Autodesk Inventor part; units mm, degrees
ref_plane "YZ Plane" through (0, 0, 0) normal (1, 0, 0) x (0, 1, 0)
ref_plane "XZ Plane" through (0, 0, 0) normal (0, 1, 0) x (-1, 0, 0)
ref_plane "XY Plane" through (0, 0, 0) normal (0, 0, 1) x (1, 0, 0)
sketch "Эскиз1" plane through (0, 0, 0) normal (0, 0, 1) x (1, 0, 0)
  circle A0 centre (-3.5, 33.9378) radius 1.5
  circle A1 centre (7, 40) radius 1.5
  circle A2 centre (-7, 40) radius 1.5
  circle A3 centre (3.5, 33.9378) radius 1.5
  arc A4 (9.6, 47.3855) -> (-9.6, 47.3855) centre (0, 18.963) ccw
  line L0 (-13, 42.6484) -> (-13, 35.2228)
  arc A5 (-12.2928, 32.6593) -> (12.2928, 32.6593) centre (0, 40) ccw
  line L1 (13, 35.2228) -> (13, 42.6484)
  circle A6 centre (0, 40) radius 3.1
  arc A7 (12.2928, 32.6593) -> (13, 35.2228) centre (8, 35.2228) ccw
  arc A8 (13, 42.6484) -> (9.6, 47.3855) centre (8, 42.6484) ccw
  arc A9 (-9.6, 47.3855) -> (-13, 42.6484) centre (-8, 42.6484) ccw
  arc A10 (-13, 35.2228) -> (-12.2928, 32.6593) centre (-8, 35.2228) ccw
  point P0 (0, 0)
extrude "Выдавливание1" add sketch "Эскиз1" against normal blind 3 contours A0 | A1 | A2 | A3
sketch "Эскиз2" plane through (7, 40, 0) normal (0, 0, 1) x (1, 0, 0)
  line L0 (6, -4.7772) -> (6, 2.6484)
  arc A0 (-19.2928, -7.3407) -> (5.2928, -7.3407) centre (-7, 0) ccw
  line L1 (-20, 2.6484) -> (-20, -4.7772)
  arc A1 (2.6, 7.3855) -> (-16.6, 7.3855) centre (-7, -21.037) ccw
  circle A2 centre (-7, 0) radius 3.1 construction
  circle A3 centre (-7, 0) radius 3.5
  arc A4 (-16.6, 7.3855) -> (-20, 2.6484) centre (-15, 2.6484) ccw
  arc A5 (6, 2.6484) -> (2.6, 7.3855) centre (1, 2.6484) ccw
  arc A6 (5.2928, -7.3407) -> (6, -4.7772) centre (1, -4.7772) ccw
  arc A7 (-20, -4.7772) -> (-19.2928, -7.3407) centre (-15, -4.7772) ccw
  point P0 (-7, -40)
  dimension "d2" = 7
extrude "Выдавливание2" add sketch "Эскиз2" along normal blind 2.8
properties part number "gasket_1"
Build history of the part. All positions in model axes, mm. A direction names the side the tool comes from. Give positions to 0.01 mm unless a question says otherwise; leave off trailing zeros. Write each loop counter-clockwise with the first axis right and the second up, starting at its lowest first coordinate (ties: lowest second). Pieces come first, ordered by that corner, then holes. Notation, with made-up numbers: (-22, 53.25) - (6, 53.25) arc R4 ccw to (6, 59.25) - close; hole circle Ø3 at (-21.75, 85.5). An arc over 180 degrees is marked (long way). Use one line per item in the form item = value. Start each with the question number.
1. 3-axis set-ups, long thin cutter, end or side, ignore diameter. For faces 4 (the face through (13, 39, 1)), 5 (the face through (6.675, 38.536, -1.479)): which of +Z, -Z, +X, -X, +Y, -Y reach the whole face in a straight line?
2. Band-saw the part on A-A on y = 40. Write the cut outline in (x, z).
3. Probe line 1 (Y direction, x = 0, z = 1.8); line 2 (Z direction, x = 0.75, y = 43.75); line 3 (Y direction, x = -1.25, z = 1.65). List the from-to ranges inside material, lowest first. Write a range as [from, to].
4. Band-saw the part on B-B on x = 0. Write the cut outline in (y, z).
5. Band-saw the part on C-C on z = 0.9. Write the cut outline in (x, y), plus the area to 3 significant figures.
6. Two-plate mould, pull along X, no slides. Class faces 1 (the face through (4.31, 35.2, -1.48)), 2 (the face through (-7, 40, -3)), 3 (the face through (12.036, 45.599, 1.38)): released by +X, released by -X, zero draft, split by the parting line, or undercut.
7. Band-saw the part on D-D on x = 7.5. Write the cut outline in (y, z).
8. Drop flat-ended pins along their axis: pin 1 Ø3 at (x, y) = (1.5, 38.5) entering from -Z; pin 2 Ø8 at (x, y) = (3, 38) entering from -Z. Give the stop position or say it passes through.
Conclusion:
q1.face_4 = +Z, -Z, +X, +Y, -Y
q1.face_5 = -Z
q2.outline = (-13, 0) - (-8.5, 0) - (-8.5, -3) - (-5.5, -3) - (-5.5, 0) - (-3.5, 0) - (-3.5, 2.8) - (-13, 2.8) - close; (3.5, 0) - (5.5, 0) - (5.5, -3) - (8.5, -3) - (8.5, 0) - (13, 0) - (13, 2.8) - (3.5, 2.8) - close
q3.line_1 = [25.68, 36.5], [43.5, 48.96]
q3.line_2 = [0, 2.8]
q3.line_3 = [25.74, 36.73], [43.27, 48.94]
q4.outline = (25.68, 0) - (36.5, 0) - (36.5, 2.8) - (25.68, 2.8) - close; (43.5, 0) - (48.96, 0) - (48.96, 2.8) - (43.5, 2.8) - close
q5.outline = (-13, 35.22) arc R5 ccw to (-12.29, 32.66) arc R14.32 ccw to (12.29, 32.66) arc R5 ccw to (13, 35.22) - (13, 42.65) arc R5 ccw to (9.6, 47.39) arc R30 ccw to (-9.6, 47.39) arc R5 ccw to (-13, 42.65) - close; hole circle Ø7 at (0, 40)
q5.area = 476 mm²
q6.face_1 = undercut
q6.face_2 = zero draft
q6.face_3 = released by +X
q7.outline = (27.8, 0) - (38.59, 0) - (38.59, -3) - (41.41, -3) - (41.41, 0) - (48.01, 0) - (48.01, 2.8) - (27.8, 2.8) - close
q8.pin_1 = 0
q8.pin_2 = -3
